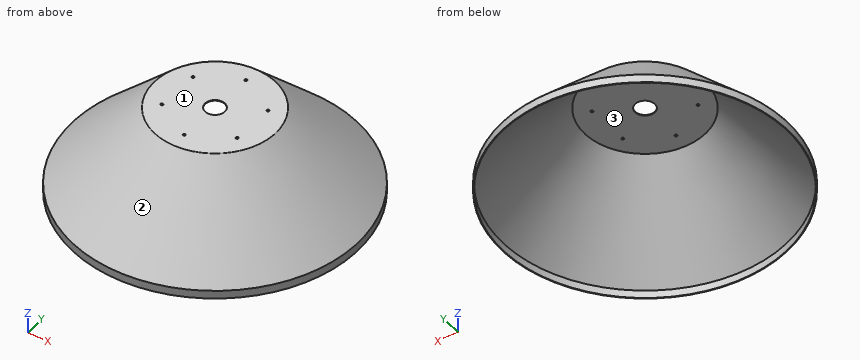
from build123d import *

# Parameters (mm, degrees)
F2_R     = 5
F3_DEPTH = 1.5
F4_R     = 20
F5_DEPTH = 179.501
F6_R     = 2.6
F7_DEPTH = 179.501


with BuildPart() as f1:
    # F0 (on Front) → F1 (revolve)
    with BuildSketch(Plane.XZ):
        with BuildLine():
            Line((288, 16), (288, 0))
            Line((288, 0), (289.5, 0))
            Line((289.5, 0), (289.5, 16.210244))
            ThreePointArc((289.5, 16.210244), (289.421822, 16.597858), (289.19951, 16.924867))
            Line((289.19951, 16.924867), (123.403494, 179.214623))
            ThreePointArc((123.403494, 179.214623), (123.081725, 179.425911), (122.703984, 179.5))
            Line((122.703984, 179.5), (0, 179.5))
            Line((0, 179.5), (0, 178))
            Line((0, 178), (122.5, 178))
            Line((122.5, 178), (288, 16))
        make_face()
    revolve(axis=Axis((0, 0, 89), (0, 0, 1)))

    # F2 (on face) → F3 (cut, through all)
    with BuildSketch(Plane.XY.offset(179.5)):
        Circle(F2_R)
    extrude(amount=-F3_DEPTH, mode=Mode.SUBTRACT)

    # F4 (on face) → F5 (cut, through all)
    with BuildSketch(Plane.XY.offset(179.5)):
        Circle(F4_R)
    extrude(amount=-F5_DEPTH, mode=Mode.SUBTRACT)

    # F6 (on face) → F7 (cut, through all)
    with BuildSketch(Plane.XY.offset(179.5)):
        with Locations((0, 89.65)):
            Circle(F6_R)
        with Locations((-77.639177, 44.825)):
            Circle(F6_R)
        with Locations((-77.639177, -44.825)):
            Circle(F6_R)
        with Locations((0, -89.65)):
            Circle(F6_R)
        with Locations((77.639177, -44.825)):
            Circle(F6_R)
        with Locations((77.639177, 44.825)):
            Circle(F6_R)
    extrude(amount=-F7_DEPTH, mode=Mode.SUBTRACT)


solid = f1.part
Geometry: final body of the model. Coordinates: model frame, mm. Face numbers are marked on the shaded views. Round coordinates to 2 decimals unless told otherwise and drop trailing zeros. Order: outer loops, then holes, each group sorted by start corner. A loop starts at its lowest first (then second) coordinate and runs counter-clockwise, first axis right, second up.
Q1. Pin query (flat end, axial travel): pin 1 (12 mm diameter, centred on x = -210, y = -161.5, fed in from -Z); pin 2 (6 mm diameter, centred on x = 77.64, y = -44.82, fed in from -Z); pin 3 (1.5 mm diameter, centred on y = 38.5, z = 121.5, fed in from +X); pin 4 (3 mm diameter, centred on x = -77.64, y = -44.82, fed in from -Z). Return the tip coordinate at first contact, or that it passes through.
Result sheet:
pin 1: stops at z = 32.72
pin 2: stops at z = 178
pin 3: stops at x = 179.05
pin 4: passes through
Q2. Section C-C, the plane z = 49. Output: boundary loops of the cut face in (x, y), and give its area (3 significant figures).
Result sheet:
outline: circle Ø512.86 at (0, 0); hole circle Ø508.57 at (0, 0)
area: 3,440 mm2
Q3. Mould query, pull axis X, two halves, no side actions, for the marked faces 1, 2 and 3. Classes: released by +X, released by -X, zero draft, split by the parting line, or undercut.
Result sheet:
face 1: zero draft
face 2: split by the parting line
face 3: undercut
Q4. Section A-A, the plane y = 0. Output: boundary loops of the cut face in (x, z).
Result sheet:
outline: (-289.5, 0) - (-288, 0) - (-288, 16) - (-122.5, 178) - (-20, 178) - (-20, 179.5) - (-122.7, 179.5) arc R1 ccw to (-123.4, 179.21) - (-289.2, 16.92) arc R1 ccw to (-289.5, 16.21) - close; (20, 178) - (122.5, 178) - (288, 16) - (288, 0) - (289.5, 0) - (289.5, 16.21) arc R1 ccw to (289.2, 16.92) - (123.4, 179.21) arc R1 ccw to (122.7, 179.5) - (20, 179.5) - close
Q5. Section B-B, the plane z = 78.5. Output: boundary loops of the cut face in (x, y).
Result sheet:
outline: circle Ø452.59 at (0, 0); hole circle Ø448.3 at (0, 0)
Q6. Material intervals for probe 1 along Y at (x, z) = (0, 178.4); probe 2 along Y at (x, z) = (0, 3); probe 3 along Z at (x, y) = (64.5, -19.5), sorted ascending.
Result sheet:
probe 1: y = -124.24 to -92.25, -87.05 to -20, 20 to 87.05, 92.25 to 124.24
probe 2: y = -289.5 to -288, 288 to 289.5
probe 3: z = 178 to 179.5
